```python
from build123d import *
from build123d.topology import SkipClean

# Parameters (mm, degrees)
ESBO_O1_R                  = 12.5
ESBO_O1_R_2                = 1.6
RESSALTO_EXTRUS_O1_DEPTH   = 10
ESBO_O3_R                  = 3.6
CORTE_EXTRUS_O1_DEPTH      = 3
RESSALTO_EXTRUS_O2_START   = 15
RESSALTO_EXTRUS_O2_DEPTH   = 15
ESBO_O4_R                  = 2.25
CORTE_EXTRUS_O2_DEPTH      = 62.613715961
ESBO_O5_R                  = 2.25
CORTE_EXTRUS_O3_DEPTH      = 51.361196938
ESBO_O6_R                  = 5
CORTE_EXTRUS_O4_DEPTH      = 3.5
ESBO_O7_R                  = 5
CORTE_EXTRUS_O5_DEPTH      = 6
ESBO_O8_R                  = 1
RESSALTO_EXTRUS_O3_DEPTH   = 5
CORTE_EXTRUS_O7_DEPTH      = 10
CORTE_EXTRUS_O7_DEPTH_BACK = 2
FILETE1_R                  = 2
CORTE_EXTRUS_O8_DEPTH      = 50.08665705
CORTE_EXTRUS_O8_DEPTH_BACK = 50.08665705


with BuildPart() as part:
    # Esboço1 → Ressalto-extrusão1 (new body)
    with BuildSketch(Plane.XY):
        Polygon((-21.50000073, 21.50000073), (-21.50000073, -21.50000073), (21.50000073, -21.50000073), (21.50000073, 38.499999791), (18.500000238, 41.49999842), (9.999999776, 41.49999842), (9.999999776, 34.324999575), (8.999999613, 34.324999575), (8.999999613, 28.674999575), (9.999999776, 28.674999575), (9.999999776, 21.50000073), align=None)
        Circle(ESBO_O1_R, mode=Mode.SUBTRACT)
        with Locations((-15.5, 15.5)):
            Circle(ESBO_O1_R_2, mode=Mode.SUBTRACT)
        with Locations((15.5, 15.5)):
            Circle(ESBO_O1_R_2, mode=Mode.SUBTRACT)
        with Locations((15.5, -15.5)):
            Circle(ESBO_O1_R_2, mode=Mode.SUBTRACT)
        with Locations((-15.5, -15.5)):
            Circle(ESBO_O1_R_2, mode=Mode.SUBTRACT)
    extrude(amount=RESSALTO_EXTRUS_O1_DEPTH)

    # Esboço3 → Corte-extrusão1 (cut)
    with BuildSketch(Plane(origin=(0, 0, 0), x_dir=(-1, 0, 0), z_dir=(0, 0, -1))):
        with Locations((-15.5, 15.5)):
            Circle(ESBO_O3_R)
        with Locations((15.5, 15.5)):
            Circle(ESBO_O3_R)
        with Locations((15.5, -15.5)):
            Circle(ESBO_O3_R)
        with Locations((-15.5, -15.5)):
            Circle(ESBO_O3_R)
    extrude(amount=-CORTE_EXTRUS_O1_DEPTH, mode=Mode.SUBTRACT)

    # Esboço2 → Ressalto-extrusão2 (add)
    with SkipClean():  # the faces are left unmerged after this step: merging them gives an invalid solid
        with BuildSketch(Plane(origin=(0, 0, 0), x_dir=(-1, 0, 0), z_dir=(0, 0, -1)).offset(RESSALTO_EXTRUS_O2_START)):
            with BuildLine():
                Line((-18.500000238, 41.49999842), (-21.50000073, 38.499999791))
                Line((-21.50000073, 38.499999791), (-21.50000073, 22.1))
                Line((-21.50000073, 22.1), (-18.50000073, 19.1))
                Line((-18.50000073, 19.1), (-15.5, 19.1))
                ThreePointArc((-15.5, 19.1), (-12.954415588, 18.045584412), (-11.9, 15.5))
                Line((-11.9, 15.5), (-11.9, 13.5))
                Line((-11.9, 13.5), (-10.9, 12.5))
                Line((-10.9, 12.5), (6.99999927, 12.5))
                Line((6.99999927, 12.5), (9.99999927, 15.5))
                Line((9.99999927, 15.5), (9.99999927, 21.50000073))
                Line((9.99999927, 21.50000073), (-9.999999776, 21.50000073))
                Line((-9.999999776, 21.50000073), (-9.999999776, 28.674999575))
                Line((-9.999999776, 28.674999575), (-8.999999613, 28.674999575))
                Line((-8.999999613, 28.674999575), (-8.999999613, 34.324999575))
                Line((-8.999999613, 34.324999575), (-9.999999776, 34.324999575))
                Line((-9.999999776, 34.324999575), (-9.999999776, 41.49999842))
                Line((-9.999999776, 41.49999842), (-18.500000238, 41.49999842))
            make_face()
        extrude(amount=-RESSALTO_EXTRUS_O2_DEPTH)

    # Esboço4 → Corte-extrusão2 (cut, through all)
    with SkipClean():  # the faces are left unmerged after this step: merging them gives an invalid solid
        with BuildSketch(Plane(origin=(21.50000073, 0, 0), x_dir=(0, 0, -1), z_dir=(1, 0, 0))):
            with Locations((2.5, 31.49999842)):
                Circle(ESBO_O4_R)
        extrude(amount=-CORTE_EXTRUS_O2_DEPTH, mode=Mode.SUBTRACT)

    # Esboço5 → Corte-extrusão3 (cut, through all)
    with SkipClean():  # the faces are left unmerged after this step: merging them gives an invalid solid
        with BuildSketch(Plane(origin=(0, 21.50000073, 0), x_dir=(1, 0, 0), z_dir=(0, 1, 0))):
            with Locations(Location((0, 7.5, 0), (0, 0, 180))):
                Circle(ESBO_O5_R)
        extrude(amount=-CORTE_EXTRUS_O3_DEPTH, mode=Mode.SUBTRACT)

    # Esboço6 → Corte-extrusão4 (cut)
    with SkipClean():  # the faces are left unmerged after this step: merging them gives an invalid solid
        with BuildSketch(Plane.XZ.offset(-12.5)):
            with Locations((0, -7.5)):
                Circle(ESBO_O6_R)
        extrude(amount=-CORTE_EXTRUS_O4_DEPTH, mode=Mode.SUBTRACT)

    # Esboço7 → Corte-extrusão5 (cut)
    with SkipClean():  # the faces are left unmerged after this step: merging them gives an invalid solid
        with BuildSketch(Plane(origin=(21.50000073, 0, 0), x_dir=(0, 0, -1), z_dir=(1, 0, 0))):
            with Locations((2.5, 31.49999842)):
                Circle(ESBO_O7_R)
        extrude(amount=-CORTE_EXTRUS_O5_DEPTH, mode=Mode.SUBTRACT)

    # Esboço8 → Ressalto-extrusão3 (add)
    with SkipClean():  # the faces are left unmerged after this step: merging them gives an invalid solid
        with BuildSketch(Plane(origin=(21.50000073, 0, 0), x_dir=(0, 0, -1), z_dir=(1, 0, 0))):
            Polygon((0, 8.49999927), (15, 8.49999927), (15, -1.50000073), (0, -1.50000073), (-2, -1.50000073), (-2, 8.49999927), align=None)
            with Locations((1.4, 3.49999927)):
                Circle(ESBO_O8_R, mode=Mode.SUBTRACT)
            with Locations((10.6, 3.49999927)):
                Circle(ESBO_O8_R, mode=Mode.SUBTRACT)
        extrude(amount=-RESSALTO_EXTRUS_O3_DEPTH)

    # Esboço9 → Corte-extrusão7 (cut, two sides: drawn at the far end of the back side and taken through both)
    with BuildSketch(Plane.ZY.offset(-16.50000073).offset(-CORTE_EXTRUS_O7_DEPTH_BACK)):
        Polygon((-9.0988893, 0.89999927), (-7.5977786, 3.49999927), (-9.0988893, 6.09999927), (-12.1011107, 6.09999927), (-13.6022214, 3.49999927), (-12.1011107, 0.89999927), align=None)
        Polygon((-4.4022214, 3.49999927), (-2.9011107, 0.89999927), (0.1011107, 0.89999927), (1.6022214, 3.49999927), (0.1011107, 6.09999927), (-2.9011107, 6.09999927), align=None)
    extrude(amount=CORTE_EXTRUS_O7_DEPTH + CORTE_EXTRUS_O7_DEPTH_BACK, mode=Mode.SUBTRACT)

    # Filete1
    filete1_edges = [part.edges().sort_by_distance(p)[0] for p in [
        (16.50000073, -0.30000073, 0),
        (19.00000073, 8.49999927, 0),
        (19.00000073, -1.50000073, 0),
        (16.50000073, 7.29999927, 0),
    ]]
    fillet(filete1_edges, radius=FILETE1_R)

    # Esboço10 → Corte-extrusão8 (cut, two sides: drawn at the far end of the back side and taken through both)
    with SkipClean():  # the faces are left unmerged after this step: merging them gives an invalid solid
        with BuildSketch(Plane(origin=(0, 0, 0), x_dir=(-1, 0, 0), z_dir=(0, 0, -1)).offset(-CORTE_EXTRUS_O8_DEPTH_BACK)):
            Polygon((-21.50000073, -3.50000073), (-19.50000073, -3.50000073), (-19.50000073, -19.50000073), (21.50000073, -19.50000073), (21.50000073, -21.50000073), (-19.50000073, -21.50000073), (-21.50000073, -21.50000073), align=None)
        extrude(amount=CORTE_EXTRUS_O8_DEPTH + CORTE_EXTRUS_O8_DEPTH_BACK, mode=Mode.SUBTRACT)


solid = part.part
```
Design review of the part built by this model. Coordinates are the model's own, in mm. A direction names the side the tool comes from. Coordinates: 2 decimals unless noted, no trailing zeros. Order: outer loops, then holes, each group sorted by start corner. A loop starts at its lowest first (then second) coordinate and runs counter-clockwise, first axis right, second up.
1) Clearance check with flat-ended pins moving along their axes: pin 1 (12 mm diameter, centred on x = -4.5, z = -3.5, fed in from -Y); pin 2 (2 mm diameter, centred on x = 14.5, y = -14.5, fed in from -Z); pin 3 (1.2 mm diameter, centred on y = 3.5, z = -10.6, fed in from +X); pin 4 (0.5 mm diameter, centred on x = 9.5, z = -2.5, fed in from +Y) (3 decimals). State where each tip first meets the part, or that it passes through.
2) Mouldability with a two-part tool opening along Z and no side actions: class faces 4 (the flat face through (17.51, 2.18, -8.36)), 5 (the cylindrical face through (15.63, -0.84, -0.35)), 6 (the flat face through (20, 40, -3)), 7 (the cylindrical face through (12.3, 33.73, -2.21)) as +Z half, -Z half, draft (parallel to the pull), parting line (faces both ways), or undercut.
3) For faces 1 (the flat face through (14.758, 4.782, 0.862)), 2 (the flat face through (-8.5, 14, -7.6)), 3 (the flat face through (2, 16, -9)), list the 3-axis set-ups (+Z, -Z, +X, -X, +Y, -Y) from which the entire face can be reached by the end or side of a thin tool; tool diameter is ignored.
4) Take a section at C-C, the plane z = 3.75. Give the boundary of the cut face in (x, y) (3 decimals), and give its area (3 significant figures).
5) Take a section at B-B, the plane x = -15.5. Give the boundary of the cut face in (y, z), and give its area (3 significant figures).
6) Take a section at D-D, the plane z = -10.6. State how many separate pieces and enclosed holes the cut face has, and give its area (3 significant figures).
7) Wall thickness on line 1 along Y through (x, z) = (18.45, -2.5); line 2 along Y through (x, z) = (-15.5, 6.25); line 3 along Y through (x, z) = (-15, 0.5): over which ranges is each line inside the solid? List them lowest first.
8) Take a section at A-A, the plane y = 0. Give the boundary of the cut face in (x, z), and give its area (3 significant figures).
Returned:
1. pin 1: stops at y = -19.5
1. pin 2: stops at z = 3
1. pin 3: passes through
1. pin 4: stops at y = 34.325
2. face 4: undercut
2. face 5: -Z half
2. face 6: draft
2. face 7: undercut
3. face 1: none
3. face 2: -Z, -X, -Y
3. face 3: -Y
4. outline: (-21.5, -19.5) - (19.5, -19.5) - (19.5, -3.5) - (21.5, -3.5) - (21.5, 38.5) - (18.5, 41.5) - (10, 41.5) - (10, 34.325) - (9, 34.325) - (9, 28.675) - (10, 28.675) - (10, 21.5) - (-21.5, 21.5) - close; hole circle Ø3.2 at (-15.5, -15.5); hole circle Ø3.2 at (-15.5, 15.5); hole circle Ø25 at (0, 0); hole circle Ø3.2 at (15.5, -15.5); hole circle Ø3.2 at (15.5, 15.5)
4. area: 1,440 mm2
5. outline: (-19.5, 0) - (-19.1, 0) - (-19.1, 3) - (-17.1, 3) - (-17.1, 10) - (-19.5, 10) - close; (-13.9, 3) - (-11.9, 3) - (-11.9, 0) - (11.9, 0) - (11.9, 3) - (13.9, 3) - (13.9, 10) - (-13.9, 10) - close; (17.1, 3) - (19.1, 3) - (19.1, 0) - (21.5, 0) - (21.5, 10) - (17.1, 10) - close
5. area: 322 mm2
6. separate pieces: 3
6. enclosed holes: 0
6. area: 451 mm2
7. line 1: y = -1.5 to 0.9, 6.1 to 8.5, 19.1 to 26.5, 36.5 to 41.5
7. line 2: y = -19.5 to -17.1, -13.9 to 13.9, 17.1 to 21.5
7. line 3: y = -19.5 to -19.07, -11.93 to 11.93, 19.07 to 21.5
8. outline: (-21.5, 0) - (-12.5, 0) - (-12.5, 10) - (-21.5, 10) - close; (12.5, 0) - (14.5, 0) arc R2 cw to (16.5, -2) - (16.5, -15) - (21.5, -15) - (21.5, 10) - (12.5, 10) - close
8. area: 256 mm2
